Read the model definition and answer for the solid it produces. Units are mm, in the model's axes. A direction names the side the tool comes from. Coordinates: 2 decimals unless noted, no trailing zeros. Write each loop counter-clockwise with the first axis right and the second up, starting at its lowest first coordinate (ties: lowest second). Pieces come first, ordered by that corner, then holes.
(1) Section C-C on z = -59 is taken. Write down the section's boundary in (x, y) (3 decimals).
(2) Section B-B on x = 23 is taken. Write down the section's boundary in (y, z) (3 decimals).
(3) Section D-D on y = 16 is taken. Write down the section's boundary in (x, z) (3 decimals), then the cut area to 3 significant figures.
(4) Section A-A on y = -4.5 is taken. Write down the section's boundary in (x, z), then the cut area to 3 significant figures.
(5) Which of the six approach directions +Z, -Z, +X, -X, +Y, -Y give full straight-line access (tool end or side, diameter ignored) to faces 1 (the flat face through (15.875, 19, -54)), 2 (the flat face through (3, -13, 6.663)), 3 (the flat face through (-25, 19, -50.487)), 4 (the flat face through (27, 0, -69.537))?
(6) Find the intervals of material crossed by probe 1 along Z at (x, y) = (-20, 10.5); probe 2 along X at (y, z) = (1, -52.5); probe 3 along Y at (x, z) = (26.5, -12) (3 decimals), in increasing order.
(7) Given pin 1 (2 mm diameter, centred on x = 1.5, z = -3, fed in from +Y) (3 decimals); pin 2 (12.5 mm diameter, centred on x = -27.5, z = -29, fed in from -Y) (3 decimals); pin 3 (5.5 mm diameter, centred on x = -31.5, y = 18.5, fed in from +Z); pin 4 (2 mm diameter, centred on y = -5.5, z = -40.5, fed in from -X), each flat-ended and moving along its own axis, determine where each tip first touches the part or whether it passes through.
(8) The mould has two halves that part along Y. Classify faces 5 (the flat face through (-21, 0, -69.525)), 6 (the flat face through (3, -11, 13.013)), 7 (the flat face through (32, 28.575, -54)): +Y half, -Y half, draft (parallel to the pull), parting line (faces both ways), or undercut.
from build123d import *

# Parameters (mm, degrees)
F0_W      = 25.4
F0_H      = 6.35
F0_W_2    = 19.05
F1_DEPTH  = 6.35
F3_DEPTH  = 6.35
F4_W      = 31.75
F4_H      = 6.35
F5_DEPTH  = 19.05
F6_W      = 41.275
F6_H      = 6.35
F7_DEPTH  = 6.35
F8_W      = 41.275
F8_H      = 6.361497178
F9_DEPTH  = 6.35
F10_W     = 6.35
F10_H     = 3.81
F11_DEPTH = 12.7


with BuildPart() as f1:
    # F0 (on Right) → F1 (new body)
    with BuildSketch(Plane.YZ):
        Polygon((-28.575, -37.7865453147), (-28.575, -31.4365453147), (-34.5734524408, -20.2424143384), (-39.0511048314, -22.6417953147), align=None)
        with Locations((-15.875, -34.6115453147)):
            Rectangle(F0_W, F0_H)
        Polygon((3.175, 25.7134546853), (-3.175, 25.7134546853), (-3.175, 13.0134546853), (-3.175, 6.6634546853), (-3.175, -31.4365453147), (-3.175, -37.7865453147), (-3.175, -75.8865453147), (3.175, -75.8865453147), align=None)
        with Locations((-12.7, 9.8384546853)):
            Rectangle(F0_W_2, F0_H)
    extrude(amount=F1_DEPTH)

    # F2 (on face) → F3 (join)
    with BuildSketch(Plane(origin=(0, 3.175, 0), x_dir=(-1, 0, 0), z_dir=(0, 1, 0))):
        Polygon((41.275, 25.7134546853), (-3.175, 25.7134546853), (-47.625, 25.7134546853), (-47.625, -75.8865453147), (-6.35, -75.8865453147), (0, -75.8865453147), (41.275, -75.8865453147), align=None)
    extrude(amount=F3_DEPTH)

    # F4 (on face) → F5 (join)
    with BuildSketch(Plane(origin=(0, 9.525, 0), x_dir=(-1, 0, 0), z_dir=(0, 1, 0))):
        with Locations((-31.75, -53.6615453147)):
            Rectangle(F4_W, F4_H)
        with Locations((25.4, -53.6615453147)):
            Rectangle(F4_W, F4_H)
    extrude(amount=F5_DEPTH)

    # F6 (on face) → F7 (join)
    with BuildSketch(Plane.XZ.offset(-3.175)):
        with Locations((26.9875, -72.7115453147)):
            Rectangle(F6_W, F6_H)
    extrude(amount=F7_DEPTH)

    # F8 (on face) → F9 (join)
    with BuildSketch(Plane.XZ.offset(-3.175)):
        with Locations((-20.6375, -72.7057967257)):
            Rectangle(F8_W, F8_H)
    extrude(amount=F9_DEPTH)

    # F10 (on face) → F11 (join)
    with BuildSketch(Plane.XY.offset(13.0134546853)):
        with Locations((3.175, -20.32)):
            Rectangle(F10_W, F10_H)
    extrude(amount=F11_DEPTH)


solid = f1.part
Response:
1. outline: (-41.275, 3.175) - (0, 3.175) - (0, -3.175) - (6.35, -3.175) - (6.35, 3.175) - (47.625, 3.175) - (47.625, 9.525) - (-41.275, 9.525) - close
2. outline: (-3.175, -75.887) - (9.525, -75.887) - (9.525, -56.837) - (28.575, -56.837) - (28.575, -50.487) - (9.525, -50.487) - (9.525, 25.713) - (3.175, 25.713) - (3.175, -69.537) - (-3.175, -69.537) - close
3. outline: (-41.275, -56.837) - (-9.525, -56.837) - (-9.525, -50.487) - (-41.275, -50.487) - close; (15.875, -56.837) - (47.625, -56.837) - (47.625, -50.487) - (15.875, -50.487) - close
3. area: 403 mm2
4. outline: (0, -37.79) - (6.35, -37.79) - (6.35, -31.44) - (0, -31.44) - close; (0, 6.66) - (6.35, 6.66) - (6.35, 13.01) - (0, 13.01) - close
4. area: 80.6 mm2
5. face 1: +Z, -Z, +Y
5. face 2: +X, -X, -Y
5. face 3: +Z, +X, -X, +Y
5. face 4: +Z, +X, -Y
6. probe 1: z = -56.84 to -50.49
6. probe 2: x = 0 to 6.35
6. probe 3: y = 3.175 to 9.525
7. pin 1: stops at y = 9.525
7. pin 2: stops at y = 3.175
7. pin 3: stops at z = -50.49
7. pin 4: passes through
8. face 5: draft
8. face 6: undercut
8. face 7: +Y half
